Check sheet for the drawn part. Datum: minimum x, y, z corner. Units: mm. Give positions to 0.01 mm unless a question says otherwise; leave off trailing zeros. Loops run counter-clockwise (first coordinate to the right, second up) from the corner with the lowest first, then second, coordinate; pieces in that order, holes last.
1. Cross-section at A-A, the plane y = 10. Record the cut outline in (x, z).
2. Cross-section at B-B, the plane x = 30. Record the cut outline in (y, z).
3. Material ranges on L1, parallel to Y at x = 10, z = 0.95; L2, parallel to X at y = 11, z = 0.9; L3, parallel to Y at x = 121.5, z = 1.3, recorded low to high.
4. Go/stop test with a flat-tipped pin: pin 1 Ø5 at (x, y) = (120, 10) entering from -Z. Record where the tip stops, or that it passes through.
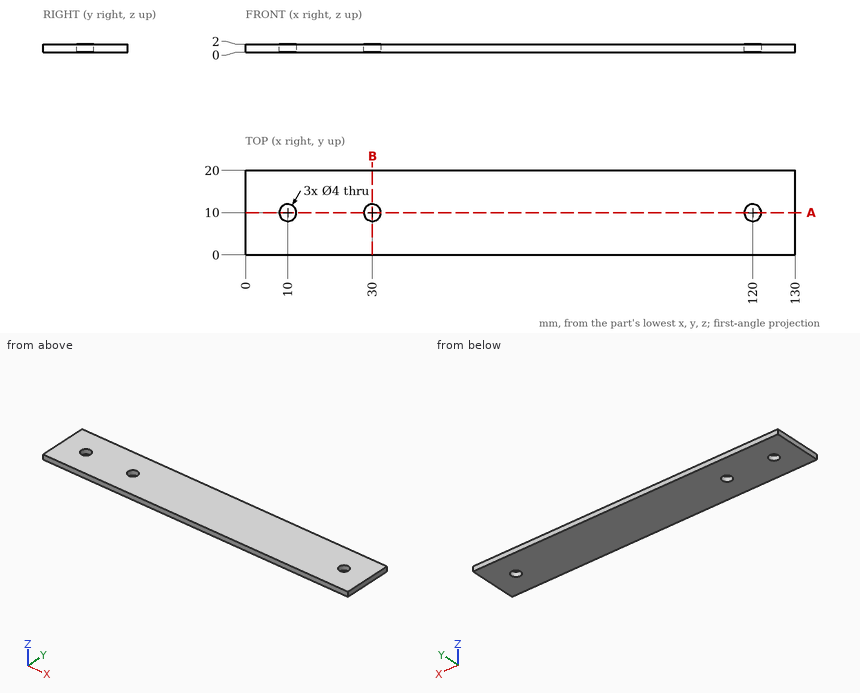
Result:
1. outline: (0, 0) - (8, 0) - (8, 2) - (0, 2) - close; (12, 0) - (28, 0) - (28, 2) - (12, 2) - close; (32, 0) - (118, 0) - (118, 2) - (32, 2) - close; (122, 0) - (130, 0) - (130, 2) - (122, 2) - close
2. outline: (0, 0) - (8, 0) - (8, 2) - (0, 2) - close; (12, 0) - (20, 0) - (20, 2) - (12, 2) - close
3. L1: y = 0 to 8, 12 to 20
3. L2: x = 0 to 8.27, 11.73 to 28.27, 31.73 to 118.27, 121.73 to 130
3. L3: y = 0 to 8.68, 11.32 to 20
4. pin 1: stops at z = 0
